Verification items for the finished model (mm, model axes). A direction names the side the tool comes from. Give positions to 0.01 mm unless a question says otherwise; leave off trailing zeros. Order: outer loops, then holes, each group sorted by start corner. A loop starts at its lowest first (then second) coordinate and runs counter-clockwise, first axis right, second up. Notation, with made-up numbers: (-39.5, 69) -> (-31.5, 69) arc R17 cw to (-31.5, 87) -> close; hole circle Ø7 at (-22.75, -32.5). An arc over 180 degrees is marked (long way). One line per question, with ' | ' between items. Start each with the question number.
Q1. Section check C-C on y = 0. Record the cut outline in (x, z).
Q2. Material ranges on probe 1 along Z at (x, y) = (2.25, 2.5); probe 2 along X at (y, z) = (0.25, 7.25); probe 3 along Y at (x, z) = (-6.5, -1.5), recorded low to high. Write a range as [from, to].
Q3. Access from +Z, -Z, +X, -X, +Y, -Y to the whole of each face (thin tool, end or side, straight path). Record for faces 1 (the flat face through (-2, -2, 0)), 2 (the flat face through (-0.53, -5.17, -1.48)).
Q4. Section check D-D on z = 4.5. Record the cut outline in (x, y), plus the area to 3 significant figures.
Q5. Section check A-A on z = -2. Record the cut outline in (x, y).
Q6. Section check B-B on x = 0. Record the cut outline in (y, z), plus the area to 3 significant figures.
Q7. Go/stop test with flat-tipped pins: pin 1 (1 mm diameter, centred on y = -3, z = 2.5, fed in from -X); pin 2 (4 mm diameter, centred on y = 3, z = 5, fed in from -X); pin 3 (5 mm diameter, centred on x = -2.5, z = 6.5, fed in from +Y); pin 4 (3 mm diameter, centred on x = -3, y = -1, fed in from +Z). Record where each tip stops, or that it passes through.
from build123d import *

# Parameters (mm, degrees)
SKETCH_1_R      = 2.4
EXTRUDE_1_DEPTH = 9
EXTRUDE_2_DEPTH = 3
FILLET_2_R      = 2
FILLET_3_R      = 2
FILLET_4_R      = 2


with BuildPart() as part:
    # 草图1 → 凸台-拉伸1 (new body)
    with BuildSketch(Plane.XY):
        Circle(SKETCH_1_R)
    extrude(amount=EXTRUDE_1_DEPTH)

    # 草图2 → 凸台-拉伸2 (add)
    with BuildSketch(Plane(origin=(0, 0, 0), x_dir=(-1, 0, 0), z_dir=(0, 0, -1))):
        Polygon((9.54506031, -4.109966384), (-1.213194857, 10.321247901), (-8.331865453, -6.211281517), align=None)
    extrude(amount=EXTRUDE_2_DEPTH)

    # 圆角2
    fillet_2_edges = [part.edges().sort_by_distance(p)[0] for p in [
        (-9.54506031, -4.109966384, -1.5),
    ]]
    fillet(fillet_2_edges, radius=FILLET_2_R)

    # 圆角3
    fillet_3_edges = [part.edges().sort_by_distance(p)[0] for p in [
        (1.213194857, 10.321247901, -1.5),
    ]]
    fillet(fillet_3_edges, radius=FILLET_3_R)

    # 圆角4
    fillet_4_edges = [part.edges().sort_by_distance(p)[0] for p in [
        (8.331865453, -6.211281517, -1.5),
    ]]
    fillet(fillet_4_edges, radius=FILLET_4_R)


solid = part.part
Filled in:
1) outline: (-6.48, -3) -> (5.66, -3) -> (5.66, 0) -> (2.4, 0) -> (2.4, 9) -> (-2.4, 9) -> (-2.4, 0) -> (-6.48, 0) -> close
2) probe 1: [-3, 0] | probe 2: [-2.39, 2.39] | probe 3: [-4.43, -0.03]
3) face 1: +Z | face 2: +Z, -Z, -X, -Y
4) outline: circle Ø4.8 at (0, 0) | area: 18.1 mm²
5) outline: (-7.47, -1.33) arc R2 ccw to (-6.1, -4.51) -> (4.89, -5.81) arc R2 ccw to (6.96, -3.03) -> (2.58, 7.14) arc R2 ccw to (-0.86, 7.54) -> close
6) outline: (-5.23, -3) -> (8.2, -3) -> (8.2, 0) -> (2.4, 0) -> (2.4, 9) -> (-2.4, 9) -> (-2.4, 0) -> (-5.23, 0) -> close | area: 83.5 mm²
7) pin 1: through | pin 2: x = -2.18 | pin 3: y = 2.4 | pin 4: z = 9
